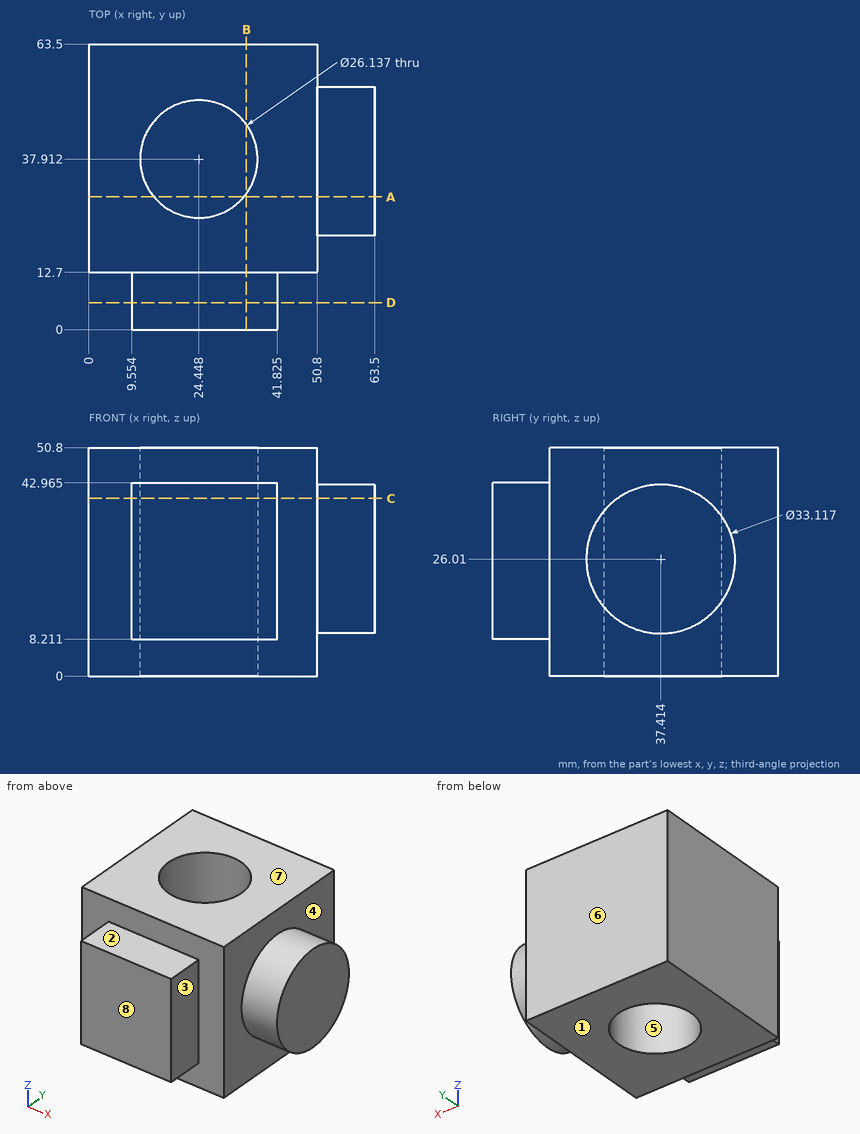
Geometry: see drawing. Coordinates: mm, zero at the bounding-box minimum. A direction names the side the tool comes from. Give positions to 0.01 mm unless a question says otherwise; leave off trailing zeros. Order: outer loops, then holes, each group sorted by start corner. A loop starts at its lowest first (then second) coordinate and runs counter-clockwise, first axis right, second up. Notation, with made-up numbers: M 48,54 L 64,54 A3 ccw 64,58 Z; hole C 59,42 d11. An arc over 180 degrees is marked long. Answer as a JSON object with one key per item and string values.
1. Ray query, line 1 (Y direction, x = 25, z = 34.5) (1 decimal); line 2 (X direction, y = 9, z = 11) (1 decimal); line 3 (X direction, y = 42, z = 45) (1 decimal). Return the intervals inside material, ascending. Write a range as [from, to].
Result sheet:
{"line 1": "[0, 24.9], [51, 63.5]", "line 2": "[9.6, 41.8]", "line 3": "[0, 12], [36.9, 50.8]"}
2. Cut plane B-B, the plane x = 35. Output: boundary loops of the cut face in (y, z) (1 decimal), and give its area (3 significant figures).
Result sheet:
{"outline": "M 0,8.2 L 12.7,8.2 L 12.7,0 L 30.2,0 L 30.2,50.8 L 12.7,50.8 L 12.7,43 L 0,43 Z; M 45.6,0 L 63.5,0 L 63.5,50.8 L 45.6,50.8 Z", "area": "2,240 mm²"}
3. Reachability of the marked faces 1, 2, 3 and 4 from +Z, -Z, +X, -X, +Y, -Y: full face, straight path, thin tool, end or side. Return the list, or none.
Result sheet:
{"face 1": "-Z, +X, -X, +Y, -Y", "face 2": "+Z, +X, -X, -Y", "face 3": "+Z, -Z, +X, -Y", "face 4": "+X"}
4. First-contact query: P1, Ø6, axis at x = 10.5, y = 38, coming from the -Z side; P2, Ø6.5, axis at y = 9.5, z = 25.5, coming from the +X side; P3, Ø14, axis at x = 30.5, y = 5.5, coming from the -Z side; P4, Ø6.5, axis at x = 19.5, y = 8.5, coming from the +Z side (1 decimal). Flat tips, straight axial feed; report the tip coordinate or a pass-through.
Result sheet:
{"P1": "z = 0", "P2": "x = 50.8", "P3": "z = 8.21", "P4": "z = 43"}
5. Pull-direction query (Y, two-part tool) for the marked faces 5, 6, 7 and 8; classes: +Y half, -Y half, draft (parallel to the pull), parting line (faces both ways), or undercut.
Result sheet:
{"face 5": "undercut", "face 6": "+Y half", "face 7": "draft", "face 8": "-Y half"}
6. Cut plane A-A, the plane y = 29.5. Output: boundary loops of the cut face in (x, z) (1 decimal), and give its area (3 significant figures).
Result sheet:
{"outline": "M 0,0 L 14.4,0 L 14.4,50.8 L 0,50.8 Z; M 34.4,0 L 50.8,0 L 50.8,11.5 L 63.5,11.5 L 63.5,40.6 L 50.8,40.6 L 50.8,50.8 L 34.4,50.8 Z", "area": "1,930 mm²"}
7. Cut plane D-D, the plane y = 6. Output: boundary loops of the cut face in (x, z) (1 decimal).
Result sheet:
{"outline": "M 9.6,8.2 L 41.8,8.2 L 41.8,43 L 9.6,43 Z"}
8. Cut plane C-C, the plane z = 39.5. Output: boundary loops of the cut face in (x, y) (1 decimal), and give its area (3 significant figures).
Result sheet:
{"outline": "M 0,12.7 L 9.6,12.7 L 9.6,0 L 41.8,0 L 41.8,12.7 L 50.8,12.7 L 50.8,27.8 L 63.5,27.8 L 63.5,47 L 50.8,47 L 50.8,63.5 L 0,63.5 Z; hole C 24.4,37.9 d26.1", "area": "2,700 mm²"}
